Verification items for the finished model (mm, model axes). Face numbers are marked on the shaded views. Round coordinates to 2 decimals unless told otherwise and drop trailing zeros. Loops run counter-clockwise (first coordinate to the right, second up) from the corner with the lowest first, then second, coordinate; pieces in that order, holes last. Notation, with made-up numbers: M 76,79 L 125,79 A26 ccw 125,101 Z; hole C 52,-33.5 d2. An arc over 180 degrees is marked long. One line per item, written item: value.
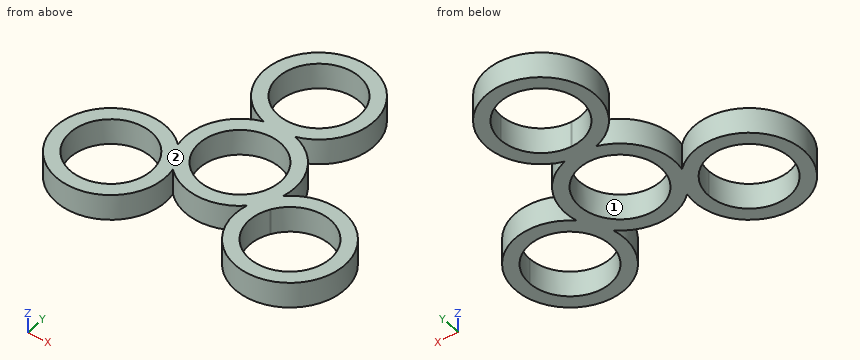
from build123d import *

# Parameters (mm, degrees)
F0_R     = 10.9982
F1_DEPTH = 7.0104
F4_DEPTH = 25.146


# Not quite as in the source:
# - a feature of the source that left no trace in its solid (it failed there, or was rolled back) is left out


with BuildPart() as f1:
    # F0 (on Top) → F1 (new body)
    with BuildSketch(Plane.XY):
        with BuildLine():
            ThreePointArc((17.2763619736, 1.5771367083), (15.0239819099, 8.6741), (10.0040214414, 14.1732))
            ThreePointArc((10.0040214414, 14.1732), (0, 45.6946), (-10.0040214414, 14.1732))
            ThreePointArc((-10.0040214414, 14.1732), (-15.0239819099, 8.6741), (-17.2763619736, 1.5771367083))
            ThreePointArc((-17.2763619736, 1.5771367083), (-39.5726844158, -22.8473), (-7.2723405322, -15.7503367083))
            ThreePointArc((-7.2723405322, -15.7503367083), (0, -17.3482), (7.2723405322, -15.7503367083))
            ThreePointArc((7.2723405322, -15.7503367083), (39.5726844158, -22.8473), (17.2763619736, 1.5771367083))
        make_face()
        with BuildLine():
            ThreePointArc((-13.5488898986, -14.1732), (-35.1543992189, -17.0912600791), (-15.0971116601, -8.5461841053))
            ThreePointArc((-15.0971116601, -8.5461841053), (-15.0225853511, -8.6732936964), (-14.9497683707, -8.8013901688))
            ThreePointArc((-14.9497683707, -8.8013901688), (-13.904869688, -11.3974658018), (-13.5488898986, -14.1732))
        make_face(mode=Mode.SUBTRACT)
        with BuildLine():
            ThreePointArc((15.0971116601, -8.5461841053), (27.466762585, -3.567503287), (35.5485151131, -14.1732))
            ThreePointArc((35.5485151131, -14.1732), (21.7729683076, -24.8170328179), (14.9497683707, -8.8013901688))
            ThreePointArc((14.9497683707, -8.8013901688), (15.0225853511, -8.6732936964), (15.0971116601, -8.5461841053))
        make_face(mode=Mode.SUBTRACT)
        Circle(F0_R, mode=Mode.SUBTRACT)
        with BuildLine():
            ThreePointArc((-0.1473432894, 17.3475742741), (-7.7257727387, 36.1763625148), (10.9998126072, 28.3464))
            ThreePointArc((10.9998126072, 28.3464), (7.8299625148, 20.6206272613), (0.1473432894, 17.3475742741))
            ThreePointArc((0.1473432894, 17.3475742741), (0, 17.3465873928), (-0.1473432894, 17.3475742741))
        make_face(mode=Mode.SUBTRACT)
    extrude(amount=F1_DEPTH)

    # F3 (on face) → F4 (cut)
    with BuildSketch(Plane(origin=(0, 0, 0), x_dir=(1, 0, 0), z_dir=(0, 0, -1))):
        with BuildLine():
            ThreePointArc((-10.0040214414, -14.1732), (0, -45.6946), (10.0040214414, -14.1732))
            ThreePointArc((10.0040214414, -14.1732), (15.0239819099, -8.6741), (17.2763619736, -1.5771367083))
            ThreePointArc((17.2763619736, -1.5771367083), (39.5726844158, 22.8473), (7.2723405322, 15.7503367083))
            ThreePointArc((7.2723405322, 15.7503367083), (0, 17.3482), (-7.2723405322, 15.7503367083))
            ThreePointArc((-7.2723405322, 15.7503367083), (-39.5726844158, 22.8473), (-17.2763619736, -1.5771367083))
            ThreePointArc((-17.2763619736, -1.5771367083), (-15.0239819099, -8.6741), (-10.0040214414, -14.1732))
        make_face()
        with BuildLine():
            ThreePointArc((10.1294026029, 10.8017600414), (37.3729807628, 21.5773005039), (14.4192999029, 3.3714399586))
            ThreePointArc((14.4192999029, 3.3714399586), (12.824278257, -7.4041005038), (4.2898973, -14.1732))
            ThreePointArc((4.2898973, -14.1732), (0, -43.1546010077), (-4.2898973, -14.1732))
            ThreePointArc((-4.2898973, -14.1732), (-12.824278257, -7.4041005038), (-14.4192999029, 3.3714399586))
            ThreePointArc((-14.4192999029, 3.3714399586), (-37.3729807628, 21.5773005038), (-10.1294026029, 10.8017600414))
            ThreePointArc((-10.1294026029, 10.8017600414), (0, 14.8082010077), (10.1294026029, 10.8017600414))
        make_face(mode=Mode.SUBTRACT)
    extrude(amount=-F4_DEPTH, mode=Mode.SUBTRACT)


solid = f1.part
(1) Sectioned sample at C-C on z = 5.5. Enter the section's corners in (x, y).
Completed:
outline: M -14.42,-3.37 A14.81 ccw long -10.13,-10.8 A14.81 ccw 10.13,-10.8 A14.81 ccw long 14.42,-3.37 A14.81 ccw 4.29,14.17 A14.81 ccw long -4.29,14.17 A14.81 ccw Z; hole C -24.55,-14.17 d22; hole C 0,0 d22; hole C 0,28.35 d22; hole C 24.55,-14.17 d22
(2) Sectioned sample at B-B on y = 10. Enter the section's corners in (x, z), and give its area (3 significant figures).
Completed:
outline: M -10.92,0 L -4.58,0 L -4.58,7.01 L -10.92,7.01 Z; M 4.58,0 L 10.92,0 L 10.92,7.01 L 4.58,7.01 Z
area: 88.9 mm^2
(3) Thickness scan on L1, parallel to Y at x = 0, z = 3.5; L2, parallel to X at y = -1, z = 2.25; L3, parallel to X at y = -20, z = 2.5. Record the ranges inside material, lowest first. Write a range as from..to.
Completed:
L1: y = -14.81..-11, 11..17.35, 39.35..43.15
L2: x = -31.31..-17.78, -14.77..-10.95, 10.95..14.77, 17.78..31.31
L3: x = -38.16..-33.88, -15.22..-10.94, 10.94..15.22, 33.88..38.16
(4) Mould release check, pull along X, two halves, no side actions. Record for the marked faces 1 and 2: +X half, -X half, draft (parallel to the pull), parting line (faces both ways), or undercut.
Completed:
face 1: undercut
face 2: draft
(5) Sectioned sample at A-A on x = 26.5. Enter the section's corners in (y, z), and give its area (3 significant figures).
Completed:
outline: M -28.85,0 L -25,0 L -25,7.01 L -28.85,7.01 Z; M -3.35,0 L 0.51,0 L 0.51,7.01 L -3.35,7.01 Z
area: 54.0 mm^2
(6) Depth check by flat-ended pin: pin 1 Ø1.5 at (y, z) = (-2.5, 3.5) entering from +X; pin 2 Ø1 at (y, z) = (13.5, 3) entering from +X; pin 3 Ø1.5 at (y, z) = (19, 5) entering from +X. Enter the tip coordinate at first touch or a pass-through.
Completed:
pin 1: stops at x = 34.55
pin 2: stops at x = 7.09
pin 3: stops at x = 12.06
